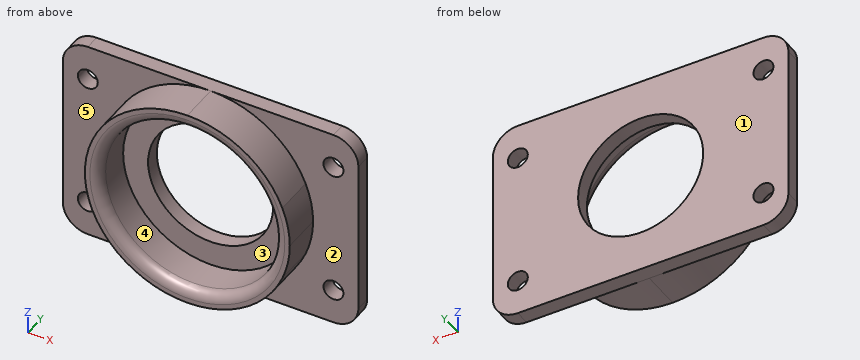
from build123d import *

# Parameters (mm, degrees)
F0_R     = 17.54425
F0_R_2   = 2
F1_DEPTH = 3
F0_R_3   = 12.54425
F2_DEPTH = 3
F3_DEPTH = 11
F4_R     = 5
F5_R     = 2


with BuildPart() as f1:
    # F0 (on Front) → F1 (new body)
    with BuildSketch(Plane.XZ):
        with BuildLine():
            ThreePointArc((19.05, 7.6917948531), (11.4900838041, 17.0306835517), (0, 20.54425))
            ThreePointArc((0, 20.54425), (-11.4900838041, 17.0306835517), (-19.05, 7.6917948531))
            Line((-19.05, 7.6917948531), (-19.05, -7.6917948531))
            ThreePointArc((-19.05, -7.6917948531), (-11.4900838386, -17.0306835284), (-8.31e-08, -20.54425))
            ThreePointArc((-8.31e-08, -20.54425), (11.4900837697, -17.0306835749), (19.05, -7.6917948531))
            Line((19.05, -7.6917948531), (19.05, 7.6917948531))
        make_face()
        Circle(F0_R, mode=Mode.SUBTRACT)
        with BuildLine():
            Line((29.6296158184, 20.54425), (19.05, 20.54425))
            Line((19.05, 20.54425), (19.05, 7.6917948531))
            ThreePointArc((19.05, 7.6917948531), (20.1672280019, 3.9177956533), (20.54425, 0))
            ThreePointArc((20.54425, 0), (20.1672280019, -3.9177956533), (19.05, -7.6917948531))
            Line((19.05, -7.6917948531), (19.05, -20.54425))
            Line((19.05, -20.54425), (29.6296158184, -20.54425))
            Line((29.6296158184, -20.54425), (29.6296158184, 20.54425))
        make_face()
        with Locations((24.6296158184, -13.4703841816)):
            Circle(F0_R_2, mode=Mode.SUBTRACT)
        with Locations((24.6296158184, 13.4703841816)):
            Circle(F0_R_2, mode=Mode.SUBTRACT)
        with BuildLine():
            Line((-19.05, 7.6917948531), (-19.05, 20.54425))
            Line((-19.05, 20.54425), (-29.6296158184, 20.54425))
            Line((-29.6296158184, 20.54425), (-29.6296158184, -20.54425))
            Line((-29.6296158184, -20.54425), (-19.05, -20.54425))
            Line((-19.05, -20.54425), (-19.05, -7.6917948531))
            ThreePointArc((-19.05, -7.6917948531), (-20.54425, 0), (-19.05, 7.6917948531))
        make_face()
        with Locations((-24.6296158184, -13.4703841816)):
            Circle(F0_R_2, mode=Mode.SUBTRACT)
        with Locations((-24.6296158184, 13.4703841816)):
            Circle(F0_R_2, mode=Mode.SUBTRACT)
        with BuildLine():
            Line((0, 20.54425), (-19.05, 20.54425))
            Line((-19.05, 20.54425), (-19.05, 7.6917948531))
            ThreePointArc((-19.05, 7.6917948531), (-11.4900838041, 17.0306835517), (0, 20.54425))
        make_face()
        with BuildLine():
            Line((-19.05, -7.6917948531), (-19.05, 7.6917948531))
            ThreePointArc((-19.05, 7.6917948531), (-20.54425, 0), (-19.05, -7.6917948531))
        make_face()
        with BuildLine():
            ThreePointArc((20.54425, 0), (20.1672280019, 3.9177956533), (19.05, 7.6917948531))
            Line((19.05, 7.6917948531), (19.05, -7.6917948531))
            ThreePointArc((19.05, -7.6917948531), (20.1672280019, -3.9177956533), (20.54425, 0))
        make_face()
        with BuildLine():
            Line((19.05, 20.54425), (0, 20.54425))
            ThreePointArc((0, 20.54425), (11.4900838041, 17.0306835517), (19.05, 7.6917948531))
            Line((19.05, 7.6917948531), (19.05, 20.54425))
        make_face()
        with BuildLine():
            Line((19.05, -20.54425), (19.05, -7.6917948531))
            ThreePointArc((19.05, -7.6917948531), (11.4900837697, -17.0306835749), (-8.31e-08, -20.54425))
            Line((-8.31e-08, -20.54425), (19.05, -20.54425))
        make_face()
        with BuildLine():
            ThreePointArc((-8.31e-08, -20.54425), (-11.4900838386, -17.0306835284), (-19.05, -7.6917948531))
            Line((-19.05, -7.6917948531), (-19.05, -20.54425))
            Line((-19.05, -20.54425), (-8.31e-08, -20.54425))
        make_face()
    extrude(amount=F1_DEPTH)

    # F0 (on Front) → F2 (join)
    with BuildSketch(Plane.XZ):
        Circle(F0_R)
        Circle(F0_R_3, mode=Mode.SUBTRACT)
    extrude(amount=F2_DEPTH)

    # F0 (on Front) → F3 (join)
    with BuildSketch(Plane.XZ):
        with BuildLine():
            ThreePointArc((19.05, 7.6917948531), (11.4900838041, 17.0306835517), (0, 20.54425))
            ThreePointArc((0, 20.54425), (-11.4900838041, 17.0306835517), (-19.05, 7.6917948531))
            Line((-19.05, 7.6917948531), (-19.05, -7.6917948531))
            ThreePointArc((-19.05, -7.6917948531), (-11.4900838386, -17.0306835284), (-8.31e-08, -20.54425))
            ThreePointArc((-8.31e-08, -20.54425), (11.4900837697, -17.0306835749), (19.05, -7.6917948531))
            Line((19.05, -7.6917948531), (19.05, 7.6917948531))
        make_face()
        Circle(F0_R, mode=Mode.SUBTRACT)
        with BuildLine():
            Line((-19.05, -7.6917948531), (-19.05, 7.6917948531))
            ThreePointArc((-19.05, 7.6917948531), (-20.54425, 0), (-19.05, -7.6917948531))
        make_face()
        with BuildLine():
            ThreePointArc((20.54425, 0), (20.1672280019, 3.9177956533), (19.05, 7.6917948531))
            Line((19.05, 7.6917948531), (19.05, -7.6917948531))
            ThreePointArc((19.05, -7.6917948531), (20.1672280019, -3.9177956533), (20.54425, 0))
        make_face()
    extrude(amount=F3_DEPTH)

    # F4
    f4_edges = [f1.edges().sort_by_distance(p)[0] for p in [
        (-29.629616, -1.5, 20.54425),
        (-29.629616, -1.5, -20.54425),
        (29.629616, -1.5, -20.54425),
        (29.629616, -1.5, 20.54425),
    ]]
    fillet(f4_edges, radius=F4_R)

    # F5
    f5_edges = [f1.edges().sort_by_distance(p)[0] for p in [
        (-17.54425, -11, 0),
    ]]
    fillet(f5_edges, radius=F5_R)


solid = f1.part
Part model, mm, in its own coordinate system. Face numbers are marked on the shaded views. A direction names the side the tool comes from. Give positions to 0.01 mm unless a question says otherwise; leave off trailing zeros. Loops run counter-clockwise (first coordinate to the right, second up) from the corner with the lowest first, then second, coordinate; pieces in that order, holes last. Notation, with made-up numbers: (18, 3) -> (40, 3) arc R24 ccw to (40, 20) -> close; hole circle Ø11 at (-32.75, 81.5). An arc over 180 degrees is marked (long way). Write each question's results on one line, items separated by ' | '. Start each with the question number.
Q1. Wall check: L1, parallel to Z at x = 0, y = -7.3; L2, parallel to Z at x = -25, y = -2.5; L3, parallel to Y at x = 10, z = 9.5. Give the ranges that are in metal, low to high.
Q2. Pin check, flat tips, straight feed: P1, Ø1.5, axis at y = -9.5, z = 16, coming from the +X side; P2, Ø3, axis at y = -7.5, z = -4, coming from the +X side; P3, Ø1.5, axis at x = 11.5, y = -7.5, coming from the -Z side. Stop position of each tip, or through.
Q3. Which spindle directions (+Z, -Z, +X, -X, +Y, -Y) get a long thin tool onto all of the face, cutting with end or side? Do the marked faces 1, 2 and 3. Say none if no direction does.
Q4. Band-saw the part on A-A on y = -5.5. List the corners of the cut face in (x, z), plus the area to 3 significant figures.
Q5. Pull direction Z, two halves, no side cores. Call the marked faces 4 and 5: +Z half, -Z half, draft (parallel to the pull), parting line (faces both ways), or undercut.
Results are:
1) L1: z = -20.54 to -17.54, 17.54 to 20.54 | L2: z = -20.53 to -15.44, -11.5 to 11.5, 15.44 to 20.53 | L3: y = -3 to 0
2) P1: stops at x = 13.77 | P2: stops at x = 20.39 | P3: stops at z = -17.51
3) face 1: +Z, -Z, +X, -X, +Y | face 2: +X, -Y | face 3: -Y
4) outline: circle Ø41.09 at (0, 0); hole circle Ø35.09 at (0, 0) | area: 359 mm²
5) face 4: undercut | face 5: draft
